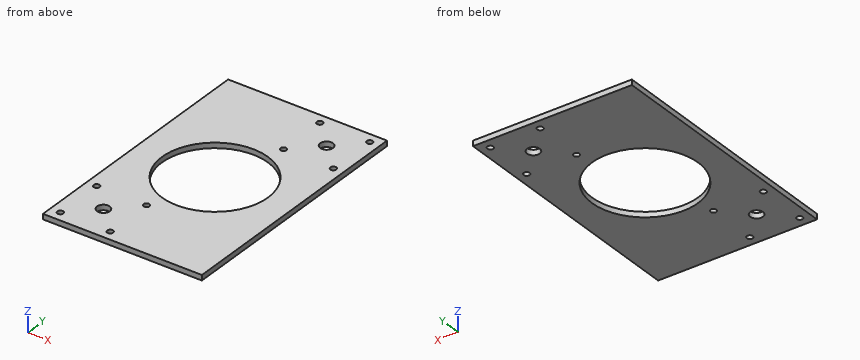
```python
from build123d import *

# Parameters (mm, degrees)
SKETCH1_W               = 150
SKETCH1_H               = 240
BOSS_EXTRUDE1_DEPTH     = 5
SKETCH7_R               = 2.8
SKETCH7_R_2             = 6
CUT_EXTRUDE4_DEPTH      = 142.598022585
SKETCH8_R               = 50
CUT_EXTRUDE5_DEPTH      = 142.598022585
DELETEFACE1_OUTLINE_R   = 6
DELETEFACE1_OUTLINE_R_2 = 2.8
DELETEFACE1_DEPTH       = 5


# Read off the part's stored shape, not the designer's step: DeleteFace1
with BuildPart() as part:
    # Sketch1 → Boss-Extrude1 (new body)
    with BuildSketch(Plane.XY):
        Rectangle(SKETCH1_W, SKETCH1_H)
    extrude(amount=BOSS_EXTRUDE1_DEPTH)

    # Sketch7 → Cut-Extrude4 (cut, through all)
    with BuildSketch(Plane.XY.offset(5)):
        with Locations((-65.55, -110.55)):
            Circle(SKETCH7_R)
        with Locations((-65.55, -63.45)):
            Circle(SKETCH7_R)
        with Locations((-18.45, -63.45)):
            Circle(SKETCH7_R)
        with Locations((-18.45, -110.55)):
            Circle(SKETCH7_R)
        with Locations(Location((-18.45, 110.55, 0), (0, 0, 180))):
            Circle(SKETCH7_R)
        with Locations(Location((-18.45, 63.45, 0), (0, 0, 180))):
            Circle(SKETCH7_R)
        with Locations(Location((-65.55, 63.45, 0), (0, 0, 180))):
            Circle(SKETCH7_R)
        with Locations(Location((-65.55, 110.55, 0), (0, 0, 180))):
            Circle(SKETCH7_R)
        with Locations((65.55, 110.55)):
            Circle(SKETCH7_R)
        with Locations((65.55, 63.45)):
            Circle(SKETCH7_R)
        with Locations((18.45, 63.45)):
            Circle(SKETCH7_R)
        with Locations((18.45, 110.55)):
            Circle(SKETCH7_R)
        with Locations(Location((18.45, -110.55, 0), (0, 0, 180))):
            Circle(SKETCH7_R)
        with Locations(Location((18.45, -63.45, 0), (0, 0, 180))):
            Circle(SKETCH7_R)
        with Locations(Location((65.55, -63.45, 0), (0, 0, 180))):
            Circle(SKETCH7_R)
        with Locations(Location((65.55, -110.55, 0), (0, 0, 180))):
            Circle(SKETCH7_R)
        with Locations((-42, -87)):
            Circle(SKETCH7_R_2)
        with Locations(Location((-42, 87, 0), (0, 0, 180))):
            Circle(SKETCH7_R_2)
        with Locations((42, 87)):
            Circle(SKETCH7_R_2)
        with Locations(Location((42, -87, 0), (0, 0, 180))):
            Circle(SKETCH7_R_2)
    extrude(amount=-CUT_EXTRUDE4_DEPTH, mode=Mode.SUBTRACT)

    # Sketch8 → Cut-Extrude5 (cut, through all)
    with BuildSketch(Plane.XY.offset(5)):
        Circle(SKETCH8_R)
    extrude(amount=-CUT_EXTRUDE5_DEPTH, mode=Mode.SUBTRACT)

    # DeleteFace1 outline → DeleteFace1 (add)
    with BuildSketch(Plane.XY):
        with Locations((42, -87)):
            Circle(DELETEFACE1_OUTLINE_R)
        with Locations((-42, 87)):
            Circle(DELETEFACE1_OUTLINE_R)
        with Locations((-65.55, 110.55)):
            Circle(DELETEFACE1_OUTLINE_R_2)
        with Locations((-65.55, 63.45)):
            Circle(DELETEFACE1_OUTLINE_R_2)
        with Locations((-18.45, 63.45)):
            Circle(DELETEFACE1_OUTLINE_R_2)
        with Locations((-18.45, 110.55)):
            Circle(DELETEFACE1_OUTLINE_R_2)
        with Locations((65.55, -110.55)):
            Circle(DELETEFACE1_OUTLINE_R_2)
        with Locations((65.55, -63.45)):
            Circle(DELETEFACE1_OUTLINE_R_2)
        with Locations((18.45, -63.45)):
            Circle(DELETEFACE1_OUTLINE_R_2)
        with Locations((18.45, -110.55)):
            Circle(DELETEFACE1_OUTLINE_R_2)
    extrude(amount=DELETEFACE1_DEPTH)


solid = part.part
```
For this review, take the finished solid that the model builds, in its own axes (mm). Coordinates: 2 decimals unless noted, no trailing zeros. Write each loop counter-clockwise with the first axis right and the second up, starting at its lowest first coordinate (ties: lowest second). Pieces come first, ordered by that corner, then holes.
(1) Wall thickness on probe 1 along Y at (x, z) = (-65.55, 3.05); probe 2 along Y at (x, z) = (-18.45, 1.5); probe 3 along Y at (x, z) = (42.5, 1.2): over which ranges is each line inside the solid? List them lowest first.
(2) Add section D-D on x = 0. Give the boundary of the cut face in (y, z).
(3) Add section A-A on x = -65.55. Give the boundary of the cut face in (y, z).
(4) Add section B-B on y = 87. Give the boundary of the cut face in (x, z), then the cut area to 3 significant figures.
(5) Add section C-C on y = -110.55. Give the boundary of the cut face in (x, z), then the cut area to 3 significant figures.
(6) For pin 1 Ø5 at (x, y) = (65.55, 63.45) entering from -Z, flat-tipped, find the tip position at first contact; note if it passes through.
Answer sheet:
1. probe 1: y = -120 to -113.35, -107.75 to -66.25, -60.65 to 120
1. probe 2: y = -120 to -113.35, -107.75 to -66.25, -60.65 to -46.47, 46.47 to 120
1. probe 3: y = -120 to -26.34, 26.34 to 81.02, 92.98 to 120
2. outline: (-120, 0) - (-50, 0) - (-50, 5) - (-120, 5) - close; (50, 0) - (120, 0) - (120, 5) - (50, 5) - close
3. outline: (-120, 0) - (-113.35, 0) - (-113.35, 5) - (-120, 5) - close; (-107.75, 0) - (-66.25, 0) - (-66.25, 5) - (-107.75, 5) - close; (-60.65, 0) - (120, 0) - (120, 5) - (-60.65, 5) - close
4. outline: (-75, 0) - (36, 0) - (36, 5) - (-75, 5) - close; (48, 0) - (75, 0) - (75, 5) - (48, 5) - close
4. area: 690 mm2
5. outline: (-75, 0) - (-68.35, 0) - (-68.35, 5) - (-75, 5) - close; (-62.75, 0) - (-21.25, 0) - (-21.25, 5) - (-62.75, 5) - close; (-15.65, 0) - (75, 0) - (75, 5) - (-15.65, 5) - close
5. area: 694 mm2
6. pin 1: passes through
